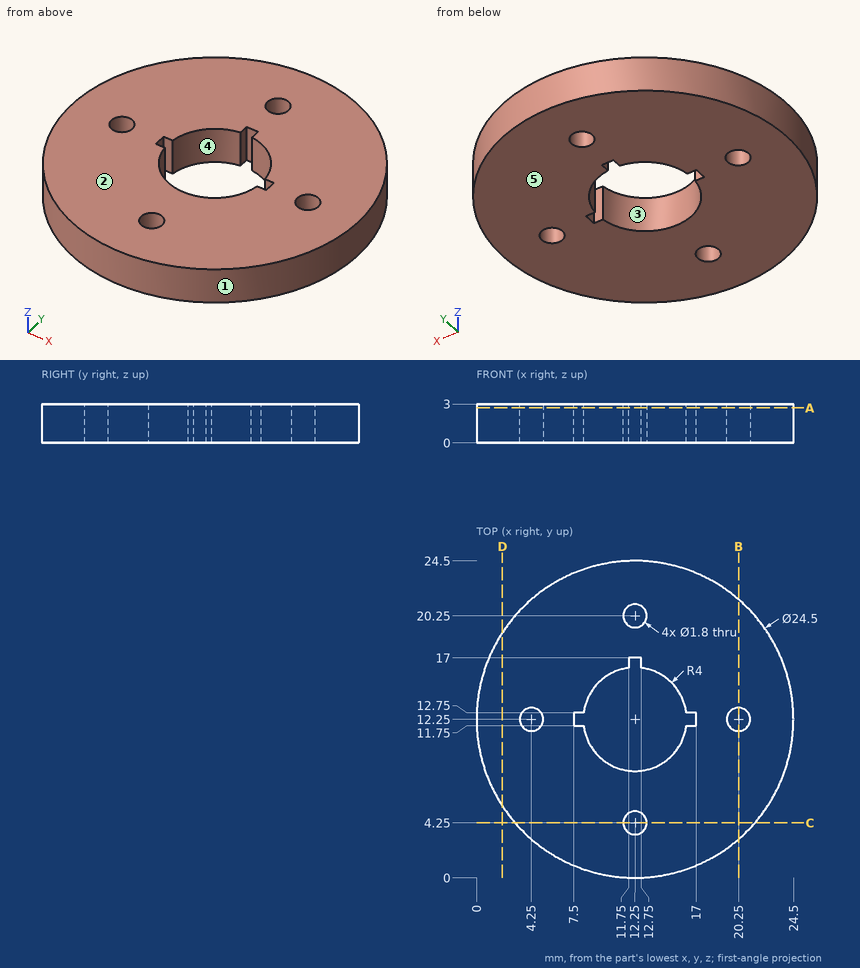
Study the drawing (mm; zero at the part's minimum x, y, z) and answer. A direction names the side the tool comes from. Coordinates: 2 decimals unless noted, no trailing zeros. Loops run counter-clockwise (first coordinate to the right, second up) from the corner with the lowest first, then second, coordinate; pieces in that order, holes last. Notation, with made-up numbers: (2, 56) -> (27, 56) arc R21 ccw to (27, 69) -> close; hole circle Ø2 at (-16.5, 0.25). An arc over 180 degrees is marked (long way). Answer in a Markdown table with one row per item. Add a question column.
1. The part is cut by section A-A, the plane z = 2.7. Write down the section's boundary in (x, y).
2. Flat-ended cylindrical pins translate along their axes: P1, Ø0.9, axis at x = 16.5, z = 1, coming from the +Y side; P2, Ø0.6, axis at x = 8, z = 2, coming from the +Y side. Find the tip coordinate at first contact, or state that the pin passes through.
3. Consider line 1 (Y direction, x = 12.25, z = 1.3); line 2 (Y direction, x = 16.25, z = 1.05); line 3 (X direction, y = 9.5, z = 2.1). Determine where each line is inside the solid, lowest interval first. Write a range as [from, to].
4. Determine the mould class of the marked faces 1, 2 and 3 for opening direction X: +X half, -X half, draft (parallel to the pull), parting line (faces both ways), or undercut.
5. For the marked faces 4 and 5, determine the directions among +Z, -Z, +X, -X, +Y, -Y from which every point of the face is accessible in a straight line to the end or side of a thin tool.
6. The part is cut by section D-D, the plane x = 2. Write down the section's boundary in (y, z), then the cut area to 3 significant figures.
7. The part is cut by section B-B, the plane x = 20.25. Write down the section's boundary in (y, z).
Answer below:
| question | item | result |
|---|---|---|
| 1 | outline | circle Ø24.5 at (12.25, 12.25); hole circle Ø1.8 at (4.25, 12.25); hole (7.5, 11.75) -> (8.28, 11.75) arc R4 ccw to (16.22, 11.75) -> (17, 11.75) -> (17, 12.75) -> (16.22, 12.75) arc R4 ccw to (12.75, 16.22) -> (12.75, 17) -> (11.75, 17) -> (11.75, 16.22) arc R4 ccw to (8.28, 12.75) -> (7.5, 12.75) -> close; hole circle Ø1.8 at (12.25, 4.25); hole circle Ø1.8 at (12.25, 20.25); hole circle Ø1.8 at (20.25, 12.25) |
| 2 | P1 | y = 23.9 |
| 2 | P2 | y = 23.85 |
| 3 | line 1 | [0, 3.35], [5.15, 8.25], [17, 19.35], [21.15, 24.5] |
| 3 | line 2 | [0.67, 11.75], [12.75, 23.83] |
| 3 | line 3 | [0.31, 9.35], [15.15, 24.19] |
| 4 | face 1 | parting line |
| 4 | face 2 | draft |
| 4 | face 3 | undercut |
| 5 | face 4 | +Z, -Z |
| 5 | face 5 | -Z, +X, -X, +Y, -Y |
| 6 | outline | (5.54, 0) -> (18.96, 0) -> (18.96, 3) -> (5.54, 3) -> close |
| 6 | area | 40.2 mm2 |
| 7 | outline | (2.97, 0) -> (11.35, 0) -> (11.35, 3) -> (2.97, 3) -> close; (13.15, 0) -> (21.53, 0) -> (21.53, 3) -> (13.15, 3) -> close |
